```python
from build123d import *

# Parameters (mm, degrees)
SKETCH_1_W          = 30.6
SKETCH_1_H          = 20.6
EXTRUDE_1_DEPTH     = 6
SKETCH_2_W          = 28.6
SKETCH_2_H          = 18.6
CUT_EXTRUDE_1_DEPTH = 4
SKETCH_3_W          = 26.6
SKETCH_3_H          = 16.6
CUT_EXTRUDE_2_DEPTH = 1
FILLET_1_R          = 2.75
FILLET_2_R          = 3.75
SKETCH_4_W          = 14.8
SKETCH_4_H          = 3
CUT_EXTRUDE_3_DEPTH = 5
FILLET_3_R          = 1.75
SKETCH_5_R          = 2.5
SKETCH_5_R_2        = 1.65
EXTRUDE_2_DEPTH     = 1
CUT_EXTRUDE_START   = -2
SKETCH_6_R          = 1.65
CUT_EXTRUDE_4_DEPTH = 2
SKETCH_7_W          = 13.8
SKETCH_7_H          = 4.8
CUT_EXTRUDE_5_DEPTH = 8
SKETCH_8_W          = 13.8
SKETCH_8_H          = 4
CUT_EXTRUDE_6_DEPTH = 10


with BuildPart() as part:
    # 草图1 → 凸台-拉伸1 (new body)
    with BuildSketch(Plane(origin=(0, 0, 0), x_dir=(1, 0, 0), z_dir=(0, 1, 0))):
        Rectangle(SKETCH_1_W, SKETCH_1_H)
    extrude(amount=EXTRUDE_1_DEPTH)

    # 草图2 → 切除-拉伸1 (cut)
    with BuildSketch(Plane(origin=(0, 6, 0), x_dir=(1, 0, 0), z_dir=(0, 1, 0))):
        Rectangle(SKETCH_2_W, SKETCH_2_H)
    extrude(amount=-CUT_EXTRUDE_1_DEPTH, mode=Mode.SUBTRACT)

    # 草图3 → 切除-拉伸2 (cut)
    with BuildSketch(Plane(origin=(0, 2, 0), x_dir=(1, 0, 0), z_dir=(0, 1, 0))):
        Rectangle(SKETCH_3_W, SKETCH_3_H)
    extrude(amount=-CUT_EXTRUDE_2_DEPTH, mode=Mode.SUBTRACT)

    # 圆角1
    fillet_1_edges = [part.edges().sort_by_distance(p)[0] for p in [
        (-14.3, 4, 9.3),
        (-14.3, 4, -9.3),
        (14.3, 4, -9.3),
        (14.3, 4, 9.3),
    ]]
    fillet(fillet_1_edges, radius=FILLET_1_R)

    # 圆角2
    fillet_2_edges = [part.edges().sort_by_distance(p)[0] for p in [
        (-15.3, 3, -10.3),
        (15.3, 3, -10.3),
        (15.3, 3, 10.3),
        (-15.3, 3, 10.3),
    ]]
    fillet(fillet_2_edges, radius=FILLET_2_R)

    # 草图4 → 切除-拉伸3 (cut)
    with BuildSketch(Plane(origin=(0, 0, -10.3), x_dir=(-1, 0, 0), z_dir=(0, 0, -1))):
        with Locations((4.9, 2.5)):
            Rectangle(SKETCH_4_W, SKETCH_4_H)
    extrude(amount=-CUT_EXTRUDE_3_DEPTH, mode=Mode.SUBTRACT)

    # 圆角3
    # the kernel refuses this fillet: 1.75 mm, written as the material it adds along each edge
    with BuildSketch(Plane(origin=(-13.3, 2, 8.3), x_dir=(1, 0, 0), z_dir=(0, -1, 0)), Plane(origin=(13.3, 2, -8.3), x_dir=(-1, 0, 0), z_dir=(0, -1, 0)), Plane(origin=(13.3, 2, 8.3), x_dir=(0, 0, -1), z_dir=(0, -1, 0))) as fillet_3_piece_1:
        with BuildLine():
            CenterArc((FILLET_3_R, -FILLET_3_R), FILLET_3_R, 90, 90)
            Line((0, -FILLET_3_R), (-FILLET_3_R * 0.02, -FILLET_3_R))
            Line((-FILLET_3_R * 0.02, -FILLET_3_R), (-FILLET_3_R * 0.02, FILLET_3_R * 0.02))
            Line((-FILLET_3_R * 0.02, FILLET_3_R * 0.02), (FILLET_3_R, FILLET_3_R * 0.02))
            Line((FILLET_3_R, FILLET_3_R * 0.02), (FILLET_3_R, 0))
        make_face()
    extrude(amount=1)
    with BuildSketch(Plane(origin=(-13.3, 2, -8.3), x_dir=(1, 0, 0), z_dir=(0, -1, 0))) as fillet_3_piece_2:
        with BuildLine():
            CenterArc((1.75, 1.58113883), FILLET_3_R, 180, 64.623066475)
            Line((0, 1.58113883), (-0.035, 1.58113883))
            Line((-0.035, 1.58113883), (-0.035, 0))
            Line((-0.035, 0), (0, -0.035))
            ThreePointArc((0, -0.035), (0.5, -0.035), (0.985, -0.031622777))
            Line((0.985, -0.031622777), (1, 0))
        make_face()
    extrude(amount=1)

    # 草图5 → 凸台-拉伸2 (add)
    # profile 1 of 2: a face of its own
    with BuildSketch(Plane(origin=(0, 1, 0), x_dir=(1, 0, 0), z_dir=(0, 1, 0))):
        with Locations((-11.25, -6.25)):
            Circle(SKETCH_5_R)
        with Locations(Location((-11.25, -6.25, 0), (0, 0, 270))):
            Circle(SKETCH_5_R_2, mode=Mode.SUBTRACT)
    # profile 2 of 2: a face of its own
    with BuildSketch(Plane(origin=(0, 1, 0), x_dir=(1, 0, 0), z_dir=(0, 1, 0))):
        with Locations((11.25, -6.25)):
            Circle(SKETCH_5_R)
        with Locations(Location((11.25, -6.25, 0), (0, 0, 270))):
            Circle(SKETCH_5_R_2, mode=Mode.SUBTRACT)
    extrude(amount=EXTRUDE_2_DEPTH)

    # 草图6 → 切除-拉伸4 (cut)
    with BuildSketch(Plane(origin=(0, 1, 0), x_dir=(1, 0, 0), z_dir=(0, 1, 0)).offset(CUT_EXTRUDE_START)):
        with Locations(Location((-11.25, -6.25, 0), (0, 0, 270))):
            Circle(SKETCH_6_R)
        with Locations(Location((11.25, -6.25, 0), (0, 0, 270))):
            Circle(SKETCH_6_R)
    extrude(amount=CUT_EXTRUDE_4_DEPTH, mode=Mode.SUBTRACT)

    # 草图7 → 切除-拉伸5 (cut)
    with BuildSketch(Plane(origin=(0, 6, 0), x_dir=(1, 0, 0), z_dir=(0, 1, 0))):
        with Locations((-1.9, -6.9)):
            Rectangle(SKETCH_7_W, SKETCH_7_H)
    extrude(amount=-CUT_EXTRUDE_5_DEPTH, mode=Mode.SUBTRACT)

    # 草图8 → 切除-拉伸6 (cut)
    with BuildSketch(Plane(origin=(0, 0, 9.3), x_dir=(-1, 0, 0), z_dir=(0, 0, -1))):
        with Locations((1.9, 4)):
            Rectangle(SKETCH_8_W, SKETCH_8_H)
    extrude(amount=-CUT_EXTRUDE_6_DEPTH, mode=Mode.SUBTRACT)


solid = part.part
```
Model file for the job. Use its own axes, mm. A direction names the side the tool comes from. Coordinates: 2 decimals unless noted, no trailing zeros. Loops run counter-clockwise (first coordinate to the right, second up) from the corner with the lowest first, then second, coordinate; pieces in that order, holes last. Notation, with made-up numbers: (72, 24.5) -> (84, 24.5) arc R30 cw to (84, 48.5) -> close; hole circle Ø11 at (41, 83). An arc over 180 degrees is marked (long way). Answer as a JSON object with one key per item and string values.
Q1. Cut at C-C (x = -11.25). List the corners of the cut face in (y, z), and give its area (4 significant figures).
Report:
{"outline": "(0, -10.3) -> (1, -10.3) -> (1, 3.75) -> (2, 3.75) -> (2, 4.6) -> (0, 4.6) -> close; (0, 7.9) -> (2, 7.9) -> (2, 9.3) -> (6, 9.3) -> (6, 10.3) -> (0, 10.3) -> close; (4, -10.3) -> (6, -10.3) -> (6, -9.3) -> (4, -9.3) -> close", "area": "26.55 mm2"}
Q2. Flat gauge pins, fed straight in: P1, Ø1, axis at x = -4.5, z = -6.5, coming from the -Y side; P2, Ø3, axis at x = -5.5, y = 4.5, coming from the +Z side; P3, Ø1, axis at y = 2, z = -9.5, coming from the -X side; P4, Ø1, axis at y = 2.5, z = -7.5, coming from the -X side. Where does each tip first touch, or does it go through?
Report:
{"P1": "stops at y = 0", "P2": "stops at z = -9.3", "P3": "stops at x = -14.39", "P4": "stops at x = -15.27"}
Q3. 3-axis set-ups, long thin cutter, end or side, ignore diameter. For faces 1 (the flat face through (-12.3, 2.1, -9.5)), 2 (the flat face through (-2, 1, 9.3)), 3 (the flat face through (-2, 2, 10)), 4 (the flat face through (-14, 2, 3)): which of +Z, -Z, +X, -X, +Y, -Y reach the whole face in a straight line?
Report:
{"face 1": "-Z", "face 2": "+Y, -Y", "face 3": "+Z, +Y", "face 4": "+Y"}
Q4. Cut at B-B (z = 6.25). List the corners of the cut face in (x, y).
Report:
{"outline": "(-15.3, 0) -> (-12.9, 0) -> (-12.9, 2) -> (-14.3, 2) -> (-14.3, 6) -> (-15.3, 6) -> close; (-9.6, 0) -> (-8.8, 0) -> (-8.8, 2) -> (-9.6, 2) -> close; (5, 0) -> (9.6, 0) -> (9.6, 2) -> (8.75, 2) -> (8.75, 1) -> (5, 1) -> close; (12.9, 0) -> (15.3, 0) -> (15.3, 6) -> (14.3, 6) -> (14.3, 2) -> (12.9, 2) -> close"}
Q5. Pull direction Z, two halves, no side cores. Call faces 5 (the flat face through (2.5, 2, -10)), 6 (the cylindrical face through (-12.25, 0.99, 4.94)), 7 (the cylindrical face through (14.172, 3.042, -9.231)), 8 (the cylindrical face through (13.52, 3.97, -8.47)): released by +Z, released by -Z, zero draft, split by the parting line, or undercut.
Report:
{"face 5": "zero draft", "face 6": "undercut", "face 7": "released by -Z", "face 8": "undercut"}
Q6. Cut at D-D (y = 3.35). List the corners of the cut face in (x, z).
Report:
{"outline": "(-15.3, -6.55) arc R3.75 ccw to (-12.3, -10.22) -> (-12.3, -9.2) arc R2.75 cw to (-14.3, -6.55) -> (-14.3, 6.55) arc R2.75 cw to (-11.55, 9.3) -> (-8.8, 9.3) -> (-8.8, 10.3) -> (-11.55, 10.3) arc R3.75 ccw to (-15.3, 6.55) -> close; (2.5, -10.3) -> (11.55, -10.3) arc R3.75 ccw to (15.3, -6.55) -> (15.3, 6.55) arc R3.75 ccw to (11.55, 10.3) -> (5, 10.3) -> (5, 9.3) -> (11.55, 9.3) arc R2.75 cw to (14.3, 6.55) -> (14.3, -6.55) arc R2.75 cw to (11.55, -9.3) -> (2.5, -9.3) -> close"}
Q7. Cut at A-A (x = 3.5). List the corners of the cut face in (y, z).
Report:
{"outline": "(0, -10.3) -> (6, -10.3) -> (6, -9.3) -> (2, -9.3) -> (2, -8.3) -> (1, -8.3) -> (1, 4.5) -> (0, 4.5) -> close; (0, 9.3) -> (2, 9.3) -> (2, 10.3) -> (0, 10.3) -> close"}
Q8. Probe probe 1 along X at (y, z) = (1.15, 6.25); probe 2 along X at (y, z) = (0.7, 6.25); probe 3 along Z at (x, y) = (11.25, 1.15). List the from-to ranges inside material, lowest first.
Report:
{"probe 1": "x = -15.3 to -12.9, -9.6 to -8.8, 8.75 to 9.6, 12.9 to 15.3", "probe 2": "x = -15.3 to -12.9, -9.6 to -8.8, 5 to 9.6, 12.9 to 15.3", "probe 3": "z = -10.3 to -8.3, 3.75 to 4.6, 7.9 to 10.3"}
